from build123d import *

# Parameters (mm, degrees)
CROQUIS1_W                  = 35
CROQUIS1_H                  = 35
SALIENTE_EXTRUIR1_DEPTH     = 0.1
CROQUIS2_R                  = 13.861230549
SALIENTE_EXTRUIR2_DEPTH     = 3
SALIENTE_EXTRUIR4_START     = 3.1
SALIENTE_EXTRUIR4_OUTLINE_R = 11.568568339
SALIENTE_EXTRUIR4_DEPTH     = 0.9
CROQUIS6_W                  = 1.5
CROQUIS6_H                  = 12
SALIENTE_EXTRUIR6_DEPTH     = 10
SALIENTE_EXTRUIR7_DEPTH     = 1.5
CROQUIS8_R                  = 1.963645542
CORTAR_EXTRUIR1_DEPTH       = 41.93570388


# Read off the part's stored shape, not the designer's step: Saliente-Extruir4
with BuildPart() as part:
    # Croquis1 → Saliente-Extruir1 (new body)
    with BuildSketch(Plane.XY):
        Rectangle(CROQUIS1_W, CROQUIS1_H)
    extrude(amount=SALIENTE_EXTRUIR1_DEPTH)

    # Croquis2 → Saliente-Extruir2 (add)
    with BuildSketch(Plane.XY.offset(0.1)):
        with Locations(Location((0, 0, 0), (0, 0, 180))):
            Circle(CROQUIS2_R)
    extrude(amount=SALIENTE_EXTRUIR2_DEPTH)

    # Saliente-Extruir4 outline → Saliente-Extruir4 (add)
    with BuildSketch(Plane.XY.offset(SALIENTE_EXTRUIR4_START)):
        Circle(SALIENTE_EXTRUIR4_OUTLINE_R)
    extrude(amount=SALIENTE_EXTRUIR4_DEPTH)

    # Croquis6 → Saliente-Extruir6 (add)
    with BuildSketch(Plane.XY.offset(4)):
        Rectangle(CROQUIS6_W, CROQUIS6_H)
    extrude(amount=SALIENTE_EXTRUIR6_DEPTH)

    # Croquis7 → Saliente-Extruir7 (add)
    with BuildSketch(Plane.ZY.offset(0.75)):
        Polygon((11.246605352, 5.859485217), (11.408857848, -6.140514783), (21.882288941, -12), (32.193467539, -5.859485217), (32.031215043, 6.140514783), (21.557783949, 12), align=None)
    extrude(amount=-SALIENTE_EXTRUIR7_DEPTH)

    # Croquis8 → Cortar-Extruir1 (cut, through all)
    with BuildSketch(Plane.ZY.offset(0.75)):
        with Locations((29.029224945, 0.140514783)):
            Circle(CROQUIS8_R)
    extrude(amount=-CORTAR_EXTRUIR1_DEPTH, mode=Mode.SUBTRACT)


solid = part.part
Design review of the part built by this model. Coordinates are the model's own, in mm. A direction names the side the tool comes from. Give positions to 0.01 mm unless a question says otherwise; leave off trailing zeros. Loops run counter-clockwise (first coordinate to the right, second up) from the corner with the lowest first, then second, coordinate; pieces in that order, holes last. Notation, with made-up numbers: M 33.25,74.25 L 70.25,74.25 A22 ccw 70.25,85.25 Z; hole C 4.5,9.25 d7. An arc over 180 degrees is marked long. One line per question, with ' | ' between items. Start each with the question number.
1. Add section C-C (x = 10.5). Write out the cut boundary in (y, z).
2. Add section D-D (z = 10). Write out the cut boundary in (x, y), plus the area to 3 significant figures.
3. Insertion check: P1, Ø8, axis at x = -5, y = -8, coming from the +Z side; P2, Ø2, axis at x = -0.5, y = -10.5, coming from the +Z side; P3, Ø1.5, axis at y = 10, z = 27.5, coming from the -X side; P4, Ø8, axis at x = 4, y = 6, coming from the +Z side. Each pin has a flat end and moves straight along its axis. Give the tip position at first contact, or say it passes through.
4. To check wall thickness, follow L1, parallel to Z at x = 8, y = -5.5; L2, parallel to X at y = -7, z = 24.5; L3, parallel to Z at x = -4.5, y = -11.5. State the ranges of each line that lie inside material, in increasing order.
5. The part is to be moulded in two halves that separate along Z. For faces 1 (the face through (-0.01, 9.03, 26.87)), 2 (the face through (0.75, 0, 18)), 3 (the face through (-0.01, 9.04, 16.59)), say which applies: released by +Z, released by -Z, zero draft, split by the parting line, or undercut.
6. For faces 4 (the face through (-0.75, 0, 18)), 5 (the face through (0, 6, 8)), 6 (the face through (0, -6, 8)), 7 (the face through (-6.396, 12.297, 1.579)), list the 3-axis set-ups (+Z, -Z, +X, -X, +Y, -Y) from which the entire face can be reached by the end or side of a thin tool; tool diameter is ignored.
7. Add section A-A (y = 1.5). Write out the cut boundary in (x, z), plus the area to 3 significant figures.
8. Add section B-B (x = 0). Write out the cut boundary in (y, z), plus the area to 3 significant figures.
Worked out:
1) outline: M -17.5,0 L 17.5,0 L 17.5,0.1 L 9.05,0.1 L 9.05,3.1 L 4.86,3.1 L 4.86,4 L -4.86,4 L -4.86,3.1 L -9.05,3.1 L -9.05,0.1 L -17.5,0.1 Z
2) outline: M -0.75,-6 L 0.75,-6 L 0.75,6 L -0.75,6 Z | area: 18.0 mm²
3) P1: stops at z = 4 | P2: stops at z = 26.08 | P3: passes through | P4: stops at z = 32.06
4) L1: z = 0 to 4 | L2: x = -0.75 to 0.75 | L3: z = 0 to 3.1
5) face 1: released by +Z | face 2: zero draft | face 3: undercut
6) face 4: +Z, -X, +Y, -Y | face 5: +X, -X, +Y | face 6: +X, -X, -Y | face 7: +Z
7) outline: M -17.5,0 L 17.5,0 L 17.5,0.1 L 13.78,0.1 L 13.78,3.1 L 11.47,3.1 L 11.47,4 L 0.75,4 L 0.75,27.61 L -0.75,27.61 L -0.75,4 L -11.47,4 L -11.47,3.1 L -13.78,3.1 L -13.78,0.1 L -17.5,0.1 Z; M -0.75,30.45 L 0.75,30.45 L 0.75,32.09 L -0.75,32.09 Z | area: 145 mm²
8) outline: M -17.5,0 L 17.5,0 L 17.5,0.1 L 13.86,0.1 L 13.86,3.1 L 11.57,3.1 L 11.57,4 L 6,4 L 6,11.48 L 12,21.56 L 6.14,32.03 L -5.86,32.19 L -12,21.88 L -6.14,11.41 L -6,11.41 L -6,4 L -11.57,4 L -11.57,3.1 L -13.86,3.1 L -13.86,0.1 L -17.5,0.1 Z; hole C 0.14,29.03 d3.93 | area: 557 mm²
